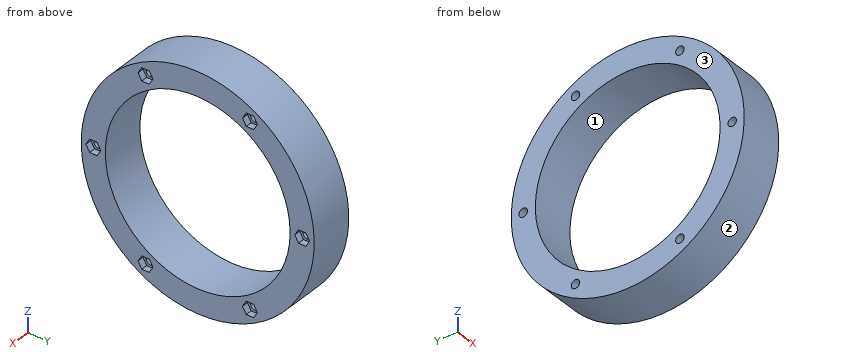
from build123d import *

# Parameters (mm, degrees)
SKETCH1_R           = 72.5
SKETCH1_R_2         = 57.5
BOSS_EXTRUDE1_DEPTH = 28
CUT_EXTRUDE1_DEPTH  = 4
CUT_EXTRUDE2_REACH  = 108.285
SKETCH3_R           = 2.65


with BuildPart() as part:
    # Sketch1 → Boss-Extrude1 (new body)
    with BuildSketch(Plane(origin=(0, 0, 0), x_dir=(0, 0, -1), z_dir=(1, 0, 0))):
        Circle(SKETCH1_R)
        Circle(SKETCH1_R_2, mode=Mode.SUBTRACT)
    extrude(amount=BOSS_EXTRUDE1_DEPTH)

    # Sketch2 → Cut-Extrude1 (cut)
    with BuildSketch(Plane(origin=(28, 0, 0), x_dir=(0, 0, -1), z_dir=(1, 0, 0))):
        Polygon((52.291651246, 30.190598923), (56.291651246, 27.881197846), (60.291651246, 30.190598923), (60.291651246, 34.809401077), (56.291651246, 37.118802154), (52.291651246, 34.809401077), align=None)
        Polygon((0, 60.381197846), (4, 62.690598923), (4, 67.309401077), (0, 69.618802154), (-4, 67.309401077), (-4, 62.690598923), align=None)
        Polygon((52.291651246, -30.190598923), (52.291651246, -34.809401077), (56.291651246, -37.118802154), (60.291651246, -34.809401077), (60.291651246, -30.190598923), (56.291651246, -27.881197846), align=None)
        Polygon((0, -60.381197846), (-4, -62.690598923), (-4, -67.309401077), (0, -69.618802154), (4, -67.309401077), (4, -62.690598923), align=None)
        Polygon((-52.291651246, -30.190598923), (-56.291651246, -27.881197846), (-60.291651246, -30.190598923), (-60.291651246, -34.809401077), (-56.291651246, -37.118802154), (-52.291651246, -34.809401077), align=None)
        Polygon((-52.291651246, 30.190598923), (-52.291651246, 34.809401077), (-56.291651246, 37.118802154), (-60.291651246, 34.809401077), (-60.291651246, 30.190598923), (-56.291651246, 27.881197846), align=None)
    extrude(amount=-CUT_EXTRUDE1_DEPTH, mode=Mode.SUBTRACT)

    # Sketch3 → Cut-Extrude2 (cut, up to next)
    with BuildSketch(Plane(origin=(28, 0, 0), x_dir=(0, 0, -1), z_dir=(1, 0, 0)), mode=Mode.PRIVATE) as cut_extrude2_sk1:
        with Locations((0, 65)):
            Circle(SKETCH3_R)
    cut_extrude2_tool1 = extrude(cut_extrude2_sk1.sketch, amount=-CUT_EXTRUDE2_REACH, mode=Mode.PRIVATE) & part.part
    # Sketch3 → Cut-Extrude2 (cut, up to next)
    with BuildSketch(Plane(origin=(28, 0, 0), x_dir=(0, 0, -1), z_dir=(1, 0, 0)), mode=Mode.PRIVATE) as cut_extrude2_sk2:
        with Locations((56.291651246, 32.5)):
            Circle(SKETCH3_R)
    cut_extrude2_tool2 = extrude(cut_extrude2_sk2.sketch, amount=-CUT_EXTRUDE2_REACH, mode=Mode.PRIVATE) & part.part
    # Sketch3 → Cut-Extrude2 (cut, up to next)
    with BuildSketch(Plane(origin=(28, 0, 0), x_dir=(0, 0, -1), z_dir=(1, 0, 0)), mode=Mode.PRIVATE) as cut_extrude2_sk3:
        with Locations((56.291651246, -32.5)):
            Circle(SKETCH3_R)
    cut_extrude2_tool3 = extrude(cut_extrude2_sk3.sketch, amount=-CUT_EXTRUDE2_REACH, mode=Mode.PRIVATE) & part.part
    # Sketch3 → Cut-Extrude2 (cut, up to next)
    with BuildSketch(Plane(origin=(28, 0, 0), x_dir=(0, 0, -1), z_dir=(1, 0, 0)), mode=Mode.PRIVATE) as cut_extrude2_sk4:
        with Locations((0, -65)):
            Circle(SKETCH3_R)
    cut_extrude2_tool4 = extrude(cut_extrude2_sk4.sketch, amount=-CUT_EXTRUDE2_REACH, mode=Mode.PRIVATE) & part.part
    # Sketch3 → Cut-Extrude2 (cut, up to next)
    with BuildSketch(Plane(origin=(28, 0, 0), x_dir=(0, 0, -1), z_dir=(1, 0, 0)), mode=Mode.PRIVATE) as cut_extrude2_sk5:
        with Locations((-56.291651246, -32.5)):
            Circle(SKETCH3_R)
    cut_extrude2_tool5 = extrude(cut_extrude2_sk5.sketch, amount=-CUT_EXTRUDE2_REACH, mode=Mode.PRIVATE) & part.part
    # Sketch3 → Cut-Extrude2 (cut, up to next)
    with BuildSketch(Plane(origin=(28, 0, 0), x_dir=(0, 0, -1), z_dir=(1, 0, 0)), mode=Mode.PRIVATE) as cut_extrude2_sk6:
        with Locations((-56.291651246, 32.5)):
            Circle(SKETCH3_R)
    cut_extrude2_tool6 = extrude(cut_extrude2_sk6.sketch, amount=-CUT_EXTRUDE2_REACH, mode=Mode.PRIVATE) & part.part
    add(cut_extrude2_tool1.solids().sort_by_distance((28, 65, 0))[0], mode=Mode.SUBTRACT)
    add(cut_extrude2_tool2.solids().sort_by_distance((28, 32.5, -56.291651))[0], mode=Mode.SUBTRACT)
    add(cut_extrude2_tool3.solids().sort_by_distance((28, -32.5, -56.291651))[0], mode=Mode.SUBTRACT)
    add(cut_extrude2_tool4.solids().sort_by_distance((28, -65, 0))[0], mode=Mode.SUBTRACT)
    add(cut_extrude2_tool5.solids().sort_by_distance((28, -32.5, 56.291651))[0], mode=Mode.SUBTRACT)
    add(cut_extrude2_tool6.solids().sort_by_distance((28, 32.5, 56.291651))[0], mode=Mode.SUBTRACT)


solid = part.part
Source: CAD feature listing. Evaluate the final solid. Frame: model axes, mm. Face numbers are marked on the shaded views. Coordinates: 2 decimals unless noted, no trailing zeros. Loops run counter-clockwise (first coordinate to the right, second up) from the corner with the lowest first, then second, coordinate; pieces in that order, holes last. Notation, with made-up numbers: (-19, 46.5) - (35, 46.5) arc R24 cw to (35, 65.5) - close; hole circle Ø4 at (-5.75, 87.5). An arc over 180 degrees is marked (long way). One line per item, written item: value. Start each with the question number.
1. Ray query, L1, parallel to Y at x = 9, z = 0; L2, parallel to Z at x = 5.75, y = 30.5; L3, parallel to Z at x = 14.25, y = 32. Return the intervals inside material, ascending.
2. Section C-C (y = -46). Return the cut outline in (x, z), and give its area (3 significant figures).
3. Section B-B (z = -9.5). Return the cut outline in (x, y), and give its area (3 significant figures).
4. Section A-A (x = 18.5). Return the cut outline in (y, z).
5. Contact query for flat-ended pins moving along their axis: P1, Ø7, axis at y = 32.5, z = -56.29, coming from the -X side; P2, Ø6, axis at x = 13.5, z = 7, coming from the -Y side; P3, Ø3, axis at x = 26.5, y = 65.5, coming from the +Z side; P4, Ø10, axis at x = 7, y = 24.5, coming from the +Z side. Output: stop coordinate, or through.
6. Section D-D (y = 32.5). Return the cut outline in (x, z).
7. Mould query, pull axis Z, two halves, no side actions, for the marked faces 1, 2 and 3. Classes: pulls with the +Z half, pulls with the -Z half, needs draft (parallel to the pull), parting line crosses it, or undercut.
Verdict:
1. L1: y = -72.5 to -67.65, -62.35 to -57.5, 57.5 to 62.35, 67.65 to 72.5
1. L2: z = -65.77 to -58.03, -54.55 to -48.74, 48.74 to 54.55, 58.03 to 65.77
1. L3: z = -65.06 to -58.89, -53.69 to -47.77, 47.77 to 53.69, 58.89 to 65.06
2. outline: (0, -56.04) - (28, -56.04) - (28, -34.5) - (0, -34.5) - close; (0, 34.5) - (28, 34.5) - (28, 56.04) - (0, 56.04) - close
2. area: 1,210 mm2
3. outline: (0, -71.87) - (28, -71.87) - (28, -56.71) - (0, -56.71) - close; (0, 56.71) - (28, 56.71) - (28, 71.87) - (0, 71.87) - close
3. area: 849 mm2
4. outline: circle Ø145 at (0, 0); hole circle Ø5.3 at (-65, 0); hole circle Ø115 at (0, 0); hole circle Ø5.3 at (-32.5, -56.29); hole circle Ø5.3 at (-32.5, 56.29); hole circle Ø5.3 at (32.5, -56.29); hole circle Ø5.3 at (32.5, 56.29); hole circle Ø5.3 at (65, 0)
5. P1: stops at x = 0
5. P2: stops at y = -72.39
5. P3: stops at z = 34.06
5. P4: stops at z = 69.83
6. outline: (0, -64.81) - (28, -64.81) - (28, -60.29) - (24, -60.29) - (24, -58.94) - (0, -58.94) - close; (0, -53.64) - (24, -53.64) - (24, -52.29) - (28, -52.29) - (28, -47.43) - (0, -47.43) - close; (0, 47.43) - (28, 47.43) - (28, 52.29) - (24, 52.29) - (24, 53.64) - (0, 53.64) - close; (0, 58.94) - (24, 58.94) - (24, 60.29) - (28, 60.29) - (28, 64.81) - (0, 64.81) - close
7. face 1: undercut
7. face 2: parting line crosses it
7. face 3: needs draft
